The listing builds one solid part. Answer for the finished solid, in the listing's coordinates (mm). A direction names the side the tool comes from. Give positions to 0.01 mm unless a question says otherwise; leave off trailing zeros. Order: outer loops, then holes, each group sorted by start corner. A loop starts at its lowest first (then second) coordinate and runs counter-clockwise, first axis right, second up.
```python
from build123d import *

# Parameters (mm, degrees)
SKETCH1_R           = 6.35
BOSS_EXTRUDE1_DEPTH = 11.049
SKETCH2_R           = 2.54
BOSS_EXTRUDE2_DEPTH = 22.86
SKETCH3_W           = 12.7
SKETCH3_H           = 5.078733264
BOSS_EXTRUDE3_DEPTH = 12.7
SKETCH4_R           = 2.3749
CUT_EXTRUDE1_DEPTH  = 12.7
FILLET2_R           = 5.08
FILLET3_R           = 5.08
FILLET5_R           = 1.27


with BuildPart() as part:
    # Sketch1 → Boss-Extrude1 (new body)
    with BuildSketch(Plane.XY):
        with Locations((-5.609264719, 0)):
            Circle(SKETCH1_R)
    extrude(amount=BOSS_EXTRUDE1_DEPTH)

    # Sketch2 → Boss-Extrude2 (add)
    with BuildSketch(Plane.XY.offset(11.049)):
        with Locations((-5.609264719, 0)):
            Circle(SKETCH2_R)
    extrude(amount=BOSS_EXTRUDE2_DEPTH)

    # Sketch3 → Boss-Extrude3 (add)
    with BuildSketch(Plane.XY.offset(33.909)):
        with Locations((-5.609264719, 0)):
            Rectangle(SKETCH3_W, SKETCH3_H)
    extrude(amount=BOSS_EXTRUDE3_DEPTH)

    # Sketch4 → Cut-Extrude1 (cut)
    with BuildSketch(Plane.XZ.offset(2.539366632)):
        with Locations(Location((-5.552545155, 40.197708747, 0), (0, 0, 270))):
            Circle(SKETCH4_R)
    extrude(amount=-CUT_EXTRUDE1_DEPTH, mode=Mode.SUBTRACT)

    # Fillet2
    fillet2_edges = [part.edges().sort_by_distance(p)[0] for p in [
        (0.740735281, 0, 46.609),
    ]]
    fillet(fillet2_edges, radius=FILLET2_R)

    # Fillet3
    fillet3_edges = [part.edges().sort_by_distance(p)[0] for p in [
        (-11.959264719, 0, 46.609),
    ]]
    fillet(fillet3_edges, radius=FILLET3_R)

    # Fillet5
    # the kernel refuses this fillet: 1.27 mm, written as the material it adds along each edge
    with BuildSketch(Plane(origin=(-5.609264719, 0, 11.049), x_dir=(1, 0, 0), z_dir=(0, -1, 0))) as fillet5_piece_1:
        with BuildLine():
            CenterArc((2.54 + FILLET5_R, FILLET5_R), FILLET5_R, 180, 90)
            Line((2.54 + FILLET5_R, 0), (2.54, 0))
            Line((2.54, 0), (2.54, FILLET5_R))
        make_face()
    revolve(axis=Axis((-5.609264719, 0, 11.049), (0, 0, 1)))
    with BuildSketch(Plane(origin=(-5.609264719, 0, 33.909), x_dir=(-0.9418707182707275, -0.3359755200370762, 0), z_dir=(-0.3359755200370762, 0.9418707182707275, 0))) as fillet5_piece_2_section:
        with BuildLine():
            CenterArc((2.54 + FILLET5_R, -FILLET5_R), FILLET5_R, 90, 90)
            Line((2.54, -FILLET5_R), (2.54, 0))
            Line((2.54, 0), (2.54 + FILLET5_R, 0))
        make_face()
    fillet5_piece_2 = revolve(axis=Axis((-5.609264719, 0, 33.909), (0, 0, 1)), revolution_arc=160.368130272, mode=Mode.PRIVATE)
    fillet5_piece_2 = split(fillet5_piece_2, bisect_by=Plane(origin=(-7.562831834, -2.539366632, 33.60366216), z_dir=(0, 1, 0)), keep=Keep.TOP, mode=Mode.PRIVATE)
    add(fillet5_piece_2)
    with BuildSketch(Plane(origin=(-5.609264719, 0, 33.909), x_dir=(0.9423620673245245, 0.3345948805164961, 0), z_dir=(0.3345948805164961, -0.9423620673245245, 0))) as fillet5_piece_3_section:
        with BuildLine():
            CenterArc((2.54 + FILLET5_R, -FILLET5_R), FILLET5_R, 90, 90)
            Line((2.54, -FILLET5_R), (2.54, 0))
            Line((2.54, 0), (2.54 + FILLET5_R, 0))
        make_face()
    fillet5_piece_3 = revolve(axis=Axis((-5.609264719, 0, 33.909), (0, 0, 1)), revolution_arc=320.904190545, mode=Mode.PRIVATE)
    fillet5_piece_3 = split(fillet5_piece_3, bisect_by=Plane(origin=(-3.654388509, -2.539366632, 33.60372255), z_dir=(0, 1, 0)), keep=Keep.TOP, mode=Mode.PRIVATE)
    fillet5_piece_3 = split(fillet5_piece_3, bisect_by=Plane(origin=(-3.654388509, 2.539366632, 33.60372255), z_dir=(0, -1, 0)), keep=Keep.TOP, mode=Mode.PRIVATE)
    add(fillet5_piece_3)
    with BuildSketch(Plane(origin=(-5.609264719, 0, 33.909), x_dir=(1, 0, 0), z_dir=(0, -1, 0))) as fillet5_piece_4_section:
        with BuildLine():
            CenterArc((2.54 + FILLET5_R, -FILLET5_R), FILLET5_R, 90, 90)
            Line((2.54, -FILLET5_R), (2.54, 0))
            Line((2.54, 0), (2.54 + FILLET5_R, 0))
        make_face()
    fillet5_piece_4 = revolve(axis=Axis((-5.609264719, 0, 33.909), (0, 0, 1)), revolution_arc=160.368130272, mode=Mode.PRIVATE)
    fillet5_piece_4 = split(fillet5_piece_4, bisect_by=Plane(origin=(-3.407688785, 2.539366632, 33.61360523), z_dir=(0, -1, 0)), keep=Keep.TOP, mode=Mode.PRIVATE)
    add(fillet5_piece_4)


solid = part.part
```
1) A tool of negligible diameter and unlimited length cuts with its end or side. For faces 4 (the cylindrical face through (0.448, 1.907, 5.447)), 5 (the cylindrical face through (-3.26, -0.97, 22.96)), 6 (the flat face through (-7, 2.539, 38)), from which of +Z, -Z, +X, -X, +Y, -Y can it reach the whole face along a straight path? Write none if from no direction.
Geometry says:
face 4: -Z
face 5: none
face 6: +Z, +X, -X, +Y
2) Find section C-C (x = -0.5). Write down the section's boundary in (y, z), then the cut area to 3 significant figures.
Geometry says:
outline: (-3.77, 0) - (3.77, 0) - (3.77, 11.05) - (-3.77, 11.05) - close; (-2.54, 33.91) - (2.54, 33.91) - (2.54, 44.86) - (-2.54, 44.86) - close
area: 139 mm2
3) Find section A-A (x = -11). Write down the section's boundary in (y, z), then the cut area to 3 significant figures.
Geometry says:
outline: (-3.36, 0) - (3.36, 0) - (3.36, 11.05) - (-3.36, 11.05) - close; (-2.54, 33.91) - (2.54, 33.91) - (2.54, 44.5) - (-2.54, 44.5) - close
area: 128 mm2
4) Straight lines are drawn through the part: probe 1 along Z at (x, y) = (-3.25, 4.5); probe 2 along Y at (x, z) = (-6.5, 43.5); probe 3 along Z at (x, y) = (-2.75, 0.5). For each, find the intervals that lie inside material, in ascending order.
Geometry says:
probe 1: z = 0 to 11.05
probe 2: y = -2.54 to 2.54
probe 3: z = 0 to 11.43, 33.53 to 46.35
5) Find section B-B (z = 24). Write down the section's boundary in (x, y), then the cut area to 3 significant figures.
Geometry says:
outline: circle Ø5.08 at (-5.61, 0)
area: 20.3 mm2
6) For a pull along Z with two mould halves and no side action, classify faces 1 (the flat face through (-11.959, 0, 38)), 2 (the flat face through (-3, -3, 11.049)), 3 (the cylindrical face through (-10.43, 0.04, 45.16)) as +Z half, -Z half, draft (parallel to the pull), parting line (faces both ways), or undercut.
Geometry says:
face 1: draft
face 2: undercut
face 3: +Z half
7) Find section D-D (y = -4.5). Write down the section's boundary in (x, z).
Geometry says:
outline: (-10.09, 0) - (-1.13, 0) - (-1.13, 11.05) - (-10.09, 11.05) - close
8) Given P1, Ø2, axis at y = -2, z = 19, coming from the +X side; P2, Ø4.5, axis at x = -5.55, z = 40.2, coming from the +Y side; P3, Ø5, axis at x = -1, z = 32.5, coming from the +Y side; P4, Ø6, axis at x = -6, z = 24, coming from the -Y side, each flat-ended and moving along its own axis, determine where each tip first touches the part or whether it passes through.
Geometry says:
P1: stops at x = -3.27
P2: passes through
P3: stops at y = 2.54
P4: stops at y = -2.54
